Autodesk Inventor part; units mm, degrees
ref_plane "YZ Plane" through (0, 0, 0) normal (1, 0, 0) x (0, 1, 0)
ref_plane "XZ Plane" through (0, 0, 0) normal (0, 1, 0) x (-1, 0, 0)
ref_plane "XY Plane" through (0, 0, 0) normal (0, 0, 1) x (1, 0, 0)
sketch "Эскиз1" plane through (0, 0, 0) normal (0, 0, 1) x (1, 0, 0)
  circle A0 centre (0, 0) radius 4.05
  line L0 (-6.05, -6.05) -> (6.05, -6.05)
  line L1 (6.05, -6.05) -> (6.05, 6.05)
  line L2 (6.05, 6.05) -> (-6.05, 6.05)
  line L3 (-6.05, 6.05) -> (-6.05, -6.05)
  line L4 (-6.05, -6.05) -> (6.05, 6.05) construction
  line L5 (6.05, -6.05) -> (-6.05, 6.05) construction
  line L6 (0, 4.05) -> (0, 6.05)
  line L7 (-4.05, 0) -> (-6.05, 0)
  line L8 (-15.15, -1.05) -> (0, -1.05)
  line L9 (0, -1.05) -> (0, -3.05)
  line L10 (0, -3.05) -> (-15.15, -3.05)
  line L11 (-15.15, -3.05) -> (-15.15, -1.05)
  line L12 (-4.05, 0) -> (4.05, 0)
  line L13 (4.05, 0) -> (4.05, -3.05)
  line L14 (4.05, -3.05) -> (-4.05, -3.05)
  line L15 (-4.05, -3.05) -> (-4.05, 0)
  line L16 (4.05, -3.05) -> (6.05, -3.05)
  line L17 (6.05, -3.05) -> (6.05, 0)
  line L18 (6.05, 0) -> (4.05, 0)
  line L19 (4.05, 0) -> (4.05, -3.05)
  point P0 (0, -2.05)
  point P1 (0, -6.05)
  point P2 (-6.05, -1.05)
  point P3 (-2.6646, -3.05)
  point P4 (-4.05, -3.05)
  point P5 (2.6646, -3.05)
  point P6 (-6.05, -3.05)
  point P7 (-4.05, -1.05)
  point P8 (-3.9115, -1.05)
  point P9 (-2.6646, -3.05)
  dimension "d0" = 8.1
  dimension "d1" = 2
  dimension "d2" = 2
  dimension "d3" = 9.1
  dimension "d4" = 2
  dimension "d5" = 3
extrude "Выдавливание1" add sketch "Эскиз1" along normal blind 1.6 contours A0 L7 L3 L2 L6 | L15 L8 L3 L7 | L15 L10 L3 L8 | L3 L10 L11 L8
sketch "Эскиз2" plane through (0, 0, 1.6) normal (0, 0, 1) x (1, 0, 0)
  line L0 (-6.05, -1.05) -> (-15.15, -1.05)
  line L1 (-15.15, -1.05) -> (-15.15, -3.05)
  line L2 (-15.15, -3.05) -> (-4.05, -3.05)
  line L3 (-4.05, -3.05) -> (-4.05, 0)
  arc A0 (0, 4.05) -> (-4.05, 0) centre (0, 0) ccw
  line L4 (0, 4.05) -> (0, 6.05)
  line L5 (0, 6.05) -> (-6.05, 6.05)
  line L6 (-6.05, 6.05) -> (-6.05, -1.05)
  line L7 (0, 4.05) -> (-4.05, 4.05)
  line L8 (-4.05, 4.05) -> (-4.05, -3.05)
  line L9 (-4.05, -3.05) -> (0, -3.05)
  line L10 (0, -3.05) -> (0, 4.05)
extrude "Выдавливание2" add sketch "Эскиз2" along normal blind 3
mirror "Зеркальное отражение1" about plane through (-9.6, -2.05, 0) normal (0, 0, -1)
sketch "Эскиз4" plane through (-15.15, -1.05, 4.6) normal (0, 1, 0) x (1, 0, 0)
  line L0 (0, 0) -> (0, 9.2)
  line L1 (0, 4.6) -> (9.1, 4.6)
  line L2 (9.1, 9.2) -> (9.1, 0)
  point P0 (15.15, 4.6)
  point P1 (4.55, 4.6)
hole "Отверстие2" at (-10.6, -1.05, 0) direction (0, -1, 0) diameter 3.2 end through all countersink diameter 6 countersink angle 90
mirror "Зеркальное отражение2" about plane through (0, 4.05, 0) normal (1, 0, 0)
sketch "Эскиз3" plane through (0, 0, 4.6) normal (0, 0, 1) x (1, 0, 0)
  arc A0 (2.6646, -3.05) -> (4.05, 0) centre (0, 0) ccw
  arc A1 (2.6646, -3.05) -> (4.05, 0) centre (0, 0) ccw
hole "Отверстие1" at (0, 0, 4.6) direction (0, 0, -1) diameter 3.5 end through all
fillet "Сопряжение1" radius 6.05 2 edges at (-6.05, 6.05, 0) (6.05, 6.05, 0)
sketch "Эскиз7" plane through (-15.15, -3.05, -4.6) normal (0, -1, 0) x (1, 0, 0)
  line L0 (30.3, 0) -> (0, 0)
  line L1 (0, 9.2) -> (30.3, 9.2)
  line L2 (13.4, 9.2) -> (16.9, 9.2)
  line L3 (15.15, 9.2) -> (15.15, 0)
  line L4 (28.3, 2) -> (2, 2)
  line L5 (2, 2) -> (2, 7.2)
  line L6 (2, 7.2) -> (28.3, 7.2)
  line L7 (28.3, 7.2) -> (28.3, 2)
  line L8 (28.3, 2) -> (2, 7.2) construction
  line L9 (2, 2) -> (28.3, 7.2) construction
  line L10 (0, 0) -> (0, 9.2)
  line L11 (30.3, 0) -> (30.3, 9.2)
  point P0 (15.15, 4.6)
  dimension "d29" = 2
  dimension "d30" = 2
extrude "Выдавливание4" add sketch "Эскиз7" along normal blind 8.25 contours L0 L3 L4 L7 L6 L1 L11 | L0 L10 L1 L3 L6 L5 L4
fillet "Сопряжение2" radius 4.55 4 edges at (15.15, -6.175, -4.6) (15.15, -6.175, 4.6) (-15.15, -6.175, -4.6) (-15.15, -6.175, 4.6)
fillet "Сопряжение3" radius 2.55 4 edges at (13.15, -7.175, -2.6) (13.15, -7.175, 2.6) (-13.15, -7.175, 2.6) (-13.15, -7.175, -2.6)
properties part number "Крышка стойки подшипника 3мм"
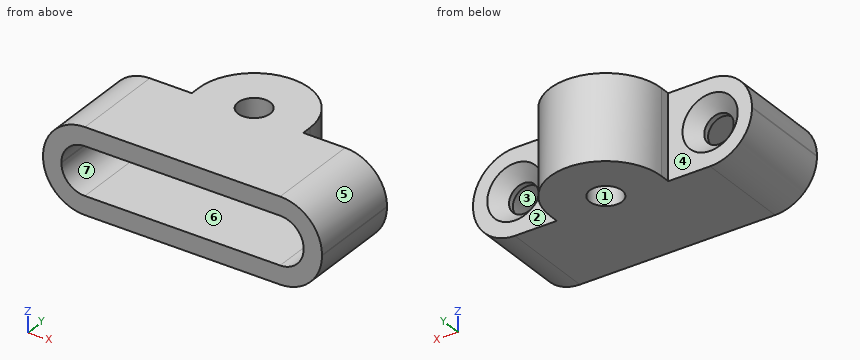
The model under review builds one solid part; all positions refer to its coordinate system, in mm. Face numbers are marked on the shaded views. A direction names the side the tool comes from. Round coordinates to 2 decimals unless told otherwise and drop trailing zeros. Order: outer loops, then holes, each group sorted by start corner. A loop starts at its lowest first (then second) coordinate and runs counter-clockwise, first axis right, second up. Notation, with made-up numbers: (18.5, 56.5) -> (31.5, 56.5) arc R19 ccw to (31.5, 70.5) -> close; hole circle Ø11 at (32.25, 34.25). An arc over 180 degrees is marked (long way). One line per item, written item: value. Start each with the question number.
Q1. Wall thickness on line 1 (X direction, y = -2.8, z = 0); line 2 (Z direction, x = 2, y = 1.75); line 3 (Z direction, x = 0, y = -7.5): over which ranges is each line inside the solid? List them lowest first.
Q2. Take a section at A-A (x = 0). Write out the cut boundary in (y, z), and give its area (3 significant figures).
Q3. Clearance check with flat-ended pins moving along their axes: pin 1 Ø0.8 at (y, z) = (-0.5, 0) entering from +X; pin 2 Ø1.6 at (x, z) = (1.5, 0) entering from -Y; pin 3 Ø0.8 at (y, z) = (-0.5, 0) entering from -X. State where each tip first meets the part, or that it passes through.
Q4. Machinability: for the marked faces 1, 2 and 3, which of the approach directions +Z, -Z, +X, -X, +Y, -Y give a long, thin tool a straight path to every point of the face, cutting with its end or side? Answer none if there is none.
Q5. Take a section at C-C (z = -3.75). Write out the cut boundary in (x, y).
Q6. Mouldability with a two-part tool opening along X and no side actions: class the marked faces 4, 5, 6 and 7 as released by +X, released by -X, zero draft, split by the parting line, or undercut.
Q7. Take a section at D-D (z = 0.75). Count the separate pieces of the cut face and the enclosed holes in it, and give its area (3 significant figures).
Q8. Take a section at B-B (y = -4.5). Write out the cut boundary in (x, z), and give its area (3 significant figures).
Reported:
1. line 1: x = -15.15 to -12.2, -9 to -4.05, 4.05 to 9, 12.2 to 15.15
1. line 2: z = -4.6 to -1.6, 1.6 to 4.6
1. line 3: z = -4.6 to -2.6, 2.6 to 4.6
2. outline: (-11.3, -4.6) -> (-1.75, -4.6) -> (-1.75, -1.6) -> (-3.05, -1.6) -> (-3.05, -2.6) -> (-11.3, -2.6) -> close; (-11.3, 2.6) -> (-3.05, 2.6) -> (-3.05, 1.6) -> (-1.75, 1.6) -> (-1.75, 4.6) -> (-11.3, 4.6) -> close; (1.75, -4.6) -> (6.05, -4.6) -> (6.05, 4.6) -> (1.75, 4.6) -> (1.75, 1.6) -> (4.05, 1.6) -> (4.05, -1.6) -> (1.75, -1.6) -> close
2. area: 73.0 mm2
3. pin 1: stops at x = 6.05
3. pin 2: stops at y = 3.33
3. pin 3: stops at x = -6.05
4. face 1: +Z, -Z
4. face 2: +Z, -Z, +X, +Y
4. face 3: -Y
5. outline: (-13.25, -11.3) -> (13.25, -11.3) -> (13.25, -1.05) -> (6.05, -1.05) -> (6.05, 0) arc R6.05 ccw to (-6.05, 0) -> (-6.05, -1.05) -> (-13.25, -1.05) -> close; hole circle Ø3.5 at (0, 0)
6. face 4: zero draft
6. face 5: released by +X
6. face 6: undercut
6. face 7: undercut
7. separate pieces: 3
7. enclosed holes: 0
7. area: 98.3 mm2
8. outline: (-15.15, -0.05) arc R4.55 ccw to (-10.6, -4.6) -> (10.6, -4.6) arc R4.55 ccw to (15.15, -0.05) -> (15.15, 0.05) arc R4.55 ccw to (10.6, 4.6) -> (-10.6, 4.6) arc R4.55 ccw to (-15.15, 0.05) -> close; hole (-13.15, -0.05) arc R2.55 ccw to (-10.6, -2.6) -> (10.6, -2.6) arc R2.55 ccw to (13.15, -0.05) -> (13.15, 0.05) arc R2.55 ccw to (10.6, 2.6) -> (-10.6, 2.6) arc R2.55 ccw to (-13.15, 0.05) -> close
8. area: 130 mm2
